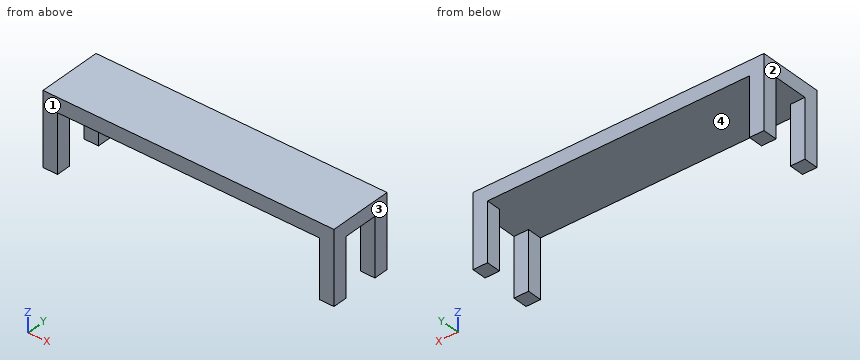
```python
from build123d import *

# Parameters (mm, degrees)
F0_W     = 254
F0_H     = 55.88
F1_DEPTH = 63.5
F2_W     = 228.6
F2_H     = 50.8
F3_DEPTH = 55.881
F4_W     = 30.48
F4_H     = 50.8
F5_DEPTH = 254.001


with BuildPart() as f1:
    # F0 (on Top) → F1 (new body)
    with BuildSketch(Plane.XY):
        with Locations((-108.656693, 13.099435)):
            Rectangle(F0_W, F0_H)
    extrude(amount=F1_DEPTH)

    # F2 (on face) → F3 (cut, through all)
    with BuildSketch(Plane.XZ.offset(14.840565)):
        with Locations((-108.656693, 25.4)):
            Rectangle(F2_W, F2_H)
    extrude(amount=-F3_DEPTH, mode=Mode.SUBTRACT)

    # F4 (on face) → F5 (cut, through all)
    with BuildSketch(Plane(origin=(-235.656693, 0, 0), x_dir=(0, -1, 0), z_dir=(-1, 0, 0))):
        with Locations((-13.099435, 25.4)):
            Rectangle(F4_W, F4_H)
    extrude(amount=-F5_DEPTH, mode=Mode.SUBTRACT)


solid = f1.part
```
Verification items for the finished model (mm, model axes). Face numbers are marked on the shaded views. Round coordinates to 2 decimals unless told otherwise and drop trailing zeros. Order: outer loops, then holes, each group sorted by start corner. A loop starts at its lowest first (then second) coordinate and runs counter-clockwise, first axis right, second up.
1) Depth check by flat-ended pin: pin 1 (3 mm diameter, centred on x = -68.5, y = 35, fed in from -Z). Enter the tip coordinate at first touch or a pass-through.
Geometry says:
pin 1: stops at z = 50.8
2) Cross-section at C-C, the plane x = -143. Record the cut outline in (y, z), plus the area to 3 significant figures.
Geometry says:
outline: (-14.84, 50.8) - (41.04, 50.8) - (41.04, 63.5) - (-14.84, 63.5) - close
area: 710 mm2
3) Cross-section at A-A, the plane z = 22.5. Record the cut outline in (x, y).
Geometry says:
outline: (-235.66, -14.84) - (-222.96, -14.84) - (-222.96, -2.14) - (-235.66, -2.14) - close; (-235.66, 28.34) - (-222.96, 28.34) - (-222.96, 41.04) - (-235.66, 41.04) - close; (5.64, -14.84) - (18.34, -14.84) - (18.34, -2.14) - (5.64, -2.14) - close; (5.64, 28.34) - (18.34, 28.34) - (18.34, 41.04) - (5.64, 41.04) - close
4) Draft check along X on the marked faces 1, 2, 3 and 4. Enter one of: +X half, -X half, draft (parallel to the pull), parting line (faces both ways), or undercut.
Geometry says:
face 1: draft
face 2: -X half
face 3: +X half
face 4: undercut
5) Cross-section at D-D, the plane y = 23. Record the cut outline in (x, z), plus the area to 3 significant figures.
Geometry says:
outline: (-235.66, 50.8) - (18.34, 50.8) - (18.34, 63.5) - (-235.66, 63.5) - close
area: 3,230 mm2
6) Material ranges on line 1 (Y direction, x = 7, z = 5); line 2 (X direction, y = -4, z = 32.5); line 3 (Z direction, x = -111, y = -6.5), recorded low to high.
Geometry says:
line 1: y = -14.84 to -2.14, 28.34 to 41.04
line 2: x = -235.66 to -222.96, 5.64 to 18.34
line 3: z = 50.8 to 63.5
7) Cross-section at B-B, the plane y = -4.5. Record the cut outline in (x, z).
Geometry says:
outline: (-235.66, 0) - (-222.96, 0) - (-222.96, 50.8) - (5.64, 50.8) - (5.64, 0) - (18.34, 0) - (18.34, 63.5) - (-235.66, 63.5) - close
